For this review, take the finished solid that the model builds, in its own axes (mm). A direction names the side the tool comes from. Coordinates: 2 decimals unless noted, no trailing zeros. Order: outer loops, then holes, each group sorted by start corner. A loop starts at its lowest first (then second) coordinate and runs counter-clockwise, first axis right, second up. Notation, with made-up numbers: (72, -34.5) - (131, -34.5) arc R33 cw to (131, 4.5) - close; hole circle Ø9 at (-6.75, 17.25). An arc over 180 degrees is marked (long way). One line per item, written item: value. Start each with the question number.
(1) Consider section A-A on y = -11. Write out the cut boundary in (x, z).
(2) Consider section D-D on y = -20.5. Write out the cut boundary in (x, z).
(3) Consider section C-C on z = 25. Write out the cut boundary in (x, y), then the cut area to 3 significant figures.
(4) To check wall thickness, follow line 1 along Z through (x, y) = (11, -54); line 2 along Y through (x, z) = (40.5, 25); line 3 along Z through (x, y) = (-73.5, -36). State the ranges of each line that lie inside material, in increasing order.
(5) Consider section B-B on x = -2. Write out the cut boundary in (y, z), then the cut area to 3 significant figures.
(6) Clearance check with flat-ended pins moving along their axes: pin 1 (6.5 mm diameter, centred on y = -65, z = 20.5, fed in from -X); pin 2 (10 mm diameter, centred on y = -35.5, z = 20, fed in from -X); pin 3 (4 mm diameter, centred on x = -29, z = 13, fed in from -Y). State where each tip first meets the part, or that it passes through.
(7) Mouldability with a two-part tool opening along Y and no side actions: class faces 5 (the flat face through (-43, -38, 14.069)), 6 (the flat face through (50, -34, 20.979)), 7 (the flat face through (-44, -50.8, 21)) as released by +Y, released by -Y, zero draft, split by the parting line, or undercut.
(8) For faces 1 (the flat face through (16.191, -64, 20)), 2 (the flat face through (25, -15, 0)), 3 (the flat face through (50, -61.594, 13)), 4 (the flat face through (-103.189, -38, 20)), list the 3-axis set-ups (+Z, -Z, +X, -X, +Y, -Y) from which the entire face can be reached by the end or side of a thin tool; tool diameter is ignored.
```python
from build123d import *

# Parameters (mm, degrees)
F0_W      = 177.8
F0_H      = 50.8
F1_DEPTH  = 76.2
F3_DEPTH  = 76.2
F4_W      = 119.38
F4_H      = 12.7
F5_DEPTH  = 25.4
F6_W      = 119.38
F6_H      = 12.7
F7_DEPTH  = 25.4
F8_W      = 62.212805
F8_H      = 35.284875
F9_DEPTH  = 25.4
F10_W     = 12.07114
F10_H     = 8.202186
F10_W_2   = 14.85679
F11_DEPTH = 25.4
F13_DEPTH = 25.4


with BuildPart() as f1:
    # F0 (on Front) → F1 (new body)
    with BuildSketch(Plane.XZ):
        with Locations((-25.930598, 9.76942)):
            Rectangle(F0_W, F0_H)
    extrude(amount=F1_DEPTH)

    # F2 (on face) → F3 (cut)
    with BuildSketch(Plane.XZ.offset(76.2)):
        Polygon((-114.830598, 35.16942), (-114.830598, -3.249923), (12.169402, -3.249923), (16.191416, 14.069194), (-103.188584, 14.069194), (-103.188584, 26.769194), (-110.808584, 26.769194), (-110.808584, 35.16942), align=None)
    extrude(amount=-F3_DEPTH, mode=Mode.SUBTRACT)

    # F4 (on face) → F5 (cut)
    with BuildSketch(Plane.XZ.offset(76.2)):
        with Locations((-43.498584, 20.419194)):
            Rectangle(F4_W, F4_H)
    extrude(amount=-F5_DEPTH, mode=Mode.SUBTRACT)

    # F6 (on face) → F7 (cut)
    with BuildSketch(Plane(origin=(0, 0, 0), x_dir=(-1, 0, 0), z_dir=(0, 1, 0))):
        with Locations((43.498584, 20.419194)):
            Rectangle(F6_W, F6_H)
    extrude(amount=-F7_DEPTH, mode=Mode.SUBTRACT)

    # F8 (on face) → F9 (cut)
    with BuildSketch(Plane.YZ.offset(62.969402)):
        with Locations((-38.844313, 9.440251)):
            Rectangle(F8_W, F8_H)
    extrude(amount=-F9_DEPTH, mode=Mode.SUBTRACT)

    # F10 (on face) → F11 (cut)
    with BuildSketch(Plane.YZ.offset(37.569402)):
        with Locations((-63.915145, -4.101093)):
            Rectangle(F10_W, F10_H)
        with Locations((-15.166305, -4.101093)):
            Rectangle(F10_W_2, F10_H)
    extrude(amount=-F11_DEPTH, mode=Mode.SUBTRACT)

    # F12 (on face) → F13 (join)
    with BuildSketch(Plane.YZ.offset(37.569402)):
        Polygon((-55.403445, 23.058975), (-61.593771, 23.058975), (-61.593771, 3.559439), (-55.403445, 3.559439), (-55.403445, 8.202186), (-52.30828, 8.202186), (-52.30828, 16.55913), (-55.403445, 16.55913), align=None)
        Polygon((-26.308898, 16.55913), (-52.30828, 16.55913), (-52.30828, 8.202186), (-47.665533, 8.202186), (-29.094545, 8.202186), (-26.308898, 8.202186), align=None)
        Polygon((-47.665533, 8.202186), (-52.30828, 8.202186), (-52.30828, 0), (-26.308898, 0), (-26.308898, 8.202186), (-29.094545, 8.202186), (-29.094545, 3.559439), (-47.665533, 3.559439), align=None)
        with BuildLine():
            ThreePointArc((-41.38843, 20.979134), (-39.308589, 18.899294), (-37.228748, 20.979134))
            Line((-37.228748, 20.979134), (-41.38843, 20.979134))
        make_face()
        with BuildLine():
            Line((-41.38843, 20.979134), (-37.228748, 20.979134))
            ThreePointArc((-37.228748, 20.979134), (-37.837919, 22.449804), (-39.308589, 23.058975))
            ThreePointArc((-39.308589, 23.058975), (-40.779258, 22.449804), (-41.38843, 20.979134))
        make_face()
        with BuildLine():
            ThreePointArc((-41.38843, 20.979134), (-40.779258, 22.449804), (-39.308589, 23.058975))
            Line((-39.308589, 23.058975), (-47.165178, 23.058975))
            Line((-47.165178, 23.058975), (-47.165178, 20.979134))
            Line((-47.165178, 20.979134), (-41.38843, 20.979134))
        make_face()
        with BuildLine():
            ThreePointArc((-39.308589, 23.058975), (-37.837919, 22.449804), (-37.228748, 20.979134))
            Line((-37.228748, 20.979134), (-30.838896, 20.979134))
            Line((-30.838896, 20.979134), (-30.838896, 23.058975))
            Line((-30.838896, 23.058975), (-39.308589, 23.058975))
        make_face()
        Polygon((-22.5947, 16.55913), (-26.308898, 16.55913), (-26.308898, 8.202186), (-22.5947, 8.202186), (-22.5947, 3.559439), (-14.237756, 3.559439), (-14.237756, 23.058975), (-22.5947, 23.058975), align=None)
    extrude(amount=F13_DEPTH)


solid = f1.part
```
Geometry check:
1. outline: (-114.83, -15.63) - (62.97, -15.63) - (62.97, -8.2) - (12.17, -8.2) - (12.17, -3.25) - (-114.83, -3.25) - close; (-110.81, 26.77) - (16.19, 26.77) - (16.19, 14.07) - (12.92, 0) - (37.57, 0) - (37.57, 27.08) - (62.97, 27.08) - (62.97, 35.17) - (-110.81, 35.17) - close
2. outline: (-114.83, -15.63) - (62.97, -15.63) - (62.97, -8.2) - (12.17, -8.2) - (12.17, -3.25) - (-114.83, -3.25) - close; (-110.81, 26.77) - (16.19, 26.77) - (16.19, 14.07) - (12.92, 0) - (37.57, 0) - (37.57, 3.56) - (62.97, 3.56) - (62.97, 23.06) - (37.57, 23.06) - (37.57, 27.08) - (62.97, 27.08) - (62.97, 35.17) - (-110.81, 35.17) - close
3. outline: (-103.19, -50.8) - (16.19, -50.8) - (16.19, -76.2) - (62.97, -76.2) - (62.97, -69.95) - (37.57, -69.95) - (37.57, -7.74) - (62.97, -7.74) - (62.97, 0) - (16.19, 0) - (16.19, -25.4) - (-103.19, -25.4) - close
3. area: 5,020 mm^2
4. line 1: z = -15.63 to -3.25, 26.77 to 35.17
4. line 2: y = -76.2 to -69.95, -7.74 to 0
4. line 3: z = -15.63 to -3.25, 14.07 to 35.17
5. outline: (-76.2, -15.63) - (0, -15.63) - (0, -3.25) - (-76.2, -3.25) - close; (-76.2, 26.77) - (-50.8, 26.77) - (-50.8, 14.07) - (-25.4, 14.07) - (-25.4, 26.77) - (0, 26.77) - (0, 35.17) - (-76.2, 35.17) - close
5. area: 1,910 mm^2
6. pin 1: stops at x = 16.19
6. pin 2: stops at x = -103.19
6. pin 3: stops at y = -50.8
7. face 5: zero draft
7. face 6: undercut
7. face 7: released by -Y
8. face 1: -X, -Y
8. face 2: +X, -X
8. face 3: +X
8. face 4: -X, +Y, -Y
